from build123d import *


with BuildPart() as f2:
    # F2: sweep along a path in F0
    with BuildLine(Plane.XZ) as f2_path:
        Line((0, 0), (-89.7624007647, 0))
        ThreePointArc((-89.7624007647, 0), (-93.4306468362, -0.6970987988), (-96.5874669216, -2.6912058481))
        ThreePointArc((-96.5874669216, -2.6912058481), (-104.9979081868, 0.8185753347), (-96.8044815522, 4.8087941519))
        ThreePointArc((-96.8044815522, 4.8087941519), (-93.8110865975, 3.0948934487), (-90.4134446565, 2.5))
        Line((-90.4134446565, 2.5), (0, 2.5))
    # F1 (on Right) → F2 (sweep)
    with BuildSketch(Plane.YZ):
        with BuildLine():
            ThreePointArc((-2.0097258966, 0), (0, -3.9869437852), (2.0097258966, 0))
            Line((2.0097258966, 0), (-2.0097258966, 0))
        make_face()
    sweep(path=f2_path.line)


solid = f2.part
Verification items for the finished model (mm, model axes). A direction names the side the tool comes from. Give positions to 0.01 mm unless a question says otherwise; leave off trailing zeros. Write each loop counter-clockwise with the first axis right and the second up, starting at its lowest first coordinate (ties: lowest second). Pieces come first, ordered by that corner, then holes. Notation, with made-up numbers: M 27,86.25 L 85,86.25 A23 ccw 85,110.25 Z; hole C 16.25,34.5 d9. An arc over 180 degrees is marked long. Write item = value, one per line.
(1) Go/stop test with flat-tipped pins: pin 1 Ø1.5 at (y, z) = (-2, 8) entering from +X; pin 2 Ø1 at (x, z) = (-17.5, -2) entering from +Y; pin 3 Ø1 at (y, z) = (2, -4.5) entering from -X; pin 4 Ø2 at (x, y) = (-67, -1) entering from -Z. Record where each tip stops, or that it passes through.
Found:
pin_1 = -94.51
pin_2 = 2.5
pin_3 = -106.64
pin_4 = -3.99
(2) Access from +Z, -Z, +X, -X, +Y, -Y to the whole of each face (thin tool, end or side, straight path). Record for faces 1 (the face through (-93.857, -0.028, 3.111)), 2 (the face through (0, 0, 5)), 3 (the face through (-45, 0, 2.5)), 4 (the face through (-44.574, 0.077, 6.486)).
Found:
face_1 = +Y, -Y
face_2 = +Z, -Z, +X, +Y, -Y
face_3 = +X, +Y, -Y
face_4 = +X
(3) Sectioned sample at B-B (y = 0). Record the cut outline in (x, z).
Found:
outline = M -96.8,4.81 A10 ccw -90.41,2.5 L 0,2.5 L 0,6.49 L -90.41,6.49 A6.01 cw -94.26,7.88 A8.99 ccw long -93.87,-5.61 A6.01 cw -89.76,-3.99 L 0,-3.99 L 0,0 L -89.76,0 A10 ccw -96.59,-2.69 A5 cw long Z
(4) Material ranges on line 1 (Z direction, x = -100, y = -0.15); line 2 (X direction, y = -0.9, z = -3.5); line 3 (X direction, y = -2, z = -1.5), recorded low to high.
Found:
line_1 = -8.02 to -4.04, 5.96 to 9.95
line_2 = -107.61 to -102.25, -97.75 to 0
line_3 = -107.6 to -104.35, -95.03 to 0
(5) Sectioned sample at A-A (x = -72.5). Record the cut outline in (y, z), then the cut area to 3 significant figures.
Found:
outline = M -2.01,0 A2.5 ccw long 2.01,0 Z; M -2.01,2.5 L 2.01,2.5 A2.5 ccw long Z
area = 33.6 mm2
(6) Draft check along Z on faces 5 (the face through (-45.51, 0.077, -3.986)), 6 (the face through (0, 0, -2)). Enter one of: released by +Z, released by -Z, zero draft, split by the parting line, or undercut.
Found:
face_5 = undercut
face_6 = zero draft
